Autodesk Inventor part; units mm, degrees
ref_plane "YZ Plane" through (0, 0, 0) normal (1, 0, 0) x (0, 1, 0)
ref_plane "XZ Plane" through (0, 0, 0) normal (0, 1, 0) x (-1, 0, 0)
ref_plane "XY Plane" through (0, 0, 0) normal (0, 0, 1) x (1, 0, 0)
sketch "Sketch1" plane through (0, 0, 0) normal (0, 1, 0) x (-1, 0, 0)
  line L0 (5, 60) -> (-5, 60)
  line L1 (-5, 60) -> (-5, -60)
  line L2 (-5, -60) -> (5, -60)
  line L3 (5, -60) -> (5, 60)
  line L4 (5, 60) -> (-5, -60) construction
  line L5 (-5, 60) -> (5, -60) construction
  point P0 (0, 0)
  dimension "d0" = 10
  dimension "d1" = 120
extrude "Extrusion1" add sketch "Sketch1" along normal blind 10
fillet "Fillet1" radius 4 4 edges at (5, 5, 60) (-5, 5, 60) (-5, 5, -60) (5, 5, -60)
sketch "Sketch2" plane through (0, 10, 0) normal (0, 1, 0) x (1, 0, 0)
  line L0 (1, 60) -> (-1, 60)
  line L1 (0, 60) -> (0, -50)
  line L2 (-1, 60) -> (-1, 55)
  arc A0 (-1, 60) -> (-5, 56) centre (-1, 56) ccw
  line L3 (-1, 55) -> (0, 55)
  point P0 (0, 0)
  dimension "d5" = 110
  dimension "d6" = 5
hole "Hole1" at (0, 10, -55) direction (0, -1, 0) diameter 4.7 depth 12
pattern_linear "Rectangular Pattern1" count 12 spacing 10 along (0, 0, 1) of "Hole1"
properties part number "soporte de direccion"
Model file for the job. Use its own axes, mm. Coordinates: 2 decimals unless noted, no trailing zeros. Loops run counter-clockwise (first coordinate to the right, second up) from the corner with the lowest first, then second, coordinate; pieces in that order, holes last. Notation, with made-up numbers: M 47,26.25 L 84,26.25 A16 cw 84,38.25 Z; hole C 55.5,63 d5. An arc over 180 degrees is marked long. Use CSV: the item, a comma, the result in double quotes. Start each with the question number.
1. Probe probe 1 along X at (y, z) = (2.75, 55); probe 2 along X at (y, z) = (6, 34); probe 3 along Z at (x, y) = (-3.5, 2.75). List the from-to ranges inside material, lowest first. Write a range as [from, to].
2. Two-plate mould, pull along X, no slides. Class faces 1 (the flat face through (-5, 5, -1)), 2 (the cylindrical face through (-0.71, 4.93, -32.76)), 3 (the cylindrical face through (3.797, 5.07, 58.859)): pulls with the +X half, pulls with the -X half, needs draft (parallel to the pull), parting line crosses it, or undercut.
3. Flat gauge pins, fed straight in: pin 1 (2 mm diameter, centred on x = 2.5, y = 5, fed in from -Z); pin 2 (5.5 mm diameter, centred on x = 0, z = 45, fed in from -Y). Where does each tip first touch, or does it go through?
4. Band-saw the part on B-B, the plane y = 5.5. Give the number of separate pieces and of enclosed holes in the cut face, then the cut area to 3 significant figures.
5. Band-saw the part on A-A, the plane z = -55. List the corners of the cut face in (x, y), then the cut area to 3 significant figures.
Entries:
1,probe 1,"x = [-5, -2.35], [2.35, 5]"
1,probe 2,"x = [-5, -2.13], [2.13, 5]"
1,probe 3,"z = [-59.12, 59.12]"
2,face 1,"pulls with the -X half"
2,face 2,"undercut"
2,face 3,"pulls with the +X half"
3,pin 1,"stops at z = -59.97"
3,pin 2,"stops at y = 0"
4,separate pieces,"1"
4,enclosed holes,"12"
4,area,"978 mm2"
5,outline,"M -5,0 L -2.35,0 L -2.35,10 L -5,10 Z; M 2.35,0 L 5,0 L 5,10 L 2.35,10 Z"
5,area,"53.0 mm2"
